Input: part model. Units: mm. Frame: model coordinates. A direction names the side the tool comes from. Round coordinates to 2 decimals unless told otherwise and drop trailing zeros. Order: outer loops, then holes, each group sorted by start corner. A loop starts at its lowest first (then second) coordinate and runs counter-clockwise, first axis right, second up. Notation, with made-up numbers: (85.5, -36.5) - (135.5, -36.5) arc R30 cw to (135.5, -0.5) - close; hole circle Ø8 at (-28.75, 16.5). An arc over 180 degrees is marked (long way). One line per item, written item: value. Start each with the question number.
Autodesk Inventor part; units mm, degrees
ref_plane "YZ Plane" through (0, 0, 0) normal (1, 0, 0) x (0, 1, 0)
ref_plane "XZ Plane" through (0, 0, 0) normal (0, 1, 0) x (-1, 0, 0)
ref_plane "XY Plane" through (0, 0, 0) normal (0, 0, 1) x (1, 0, 0)
sketch "Sketch1" plane through (0, 0, 0) normal (0, 0, 1) x (1, 0, 0)
  line L0 (20.5, -20.5) -> (20.5, -28.5)
  line L1 (28.5, -20.5) -> (20.5, -20.5)
  line L2 (28.5, 20.5) -> (28.5, -20.5)
  line L3 (20.5, 20.5) -> (28.5, 20.5)
  line L4 (20.5, 28.5) -> (20.5, 20.5)
  line L5 (-20.5, 28.5) -> (20.5, 28.5)
  line L6 (-20.5, 20.5) -> (-20.5, 28.5)
  line L7 (-28.5, 20.5) -> (-20.5, 20.5)
  line L8 (-28.5, -20.5) -> (-28.5, 20.5)
  line L9 (-20.5, -20.5) -> (-28.5, -20.5)
  line L10 (-20.5, -28.5) -> (-20.5, -20.5)
  line L11 (20.5, -28.5) -> (-20.5, -28.5)
  line L12 (-100, -100) -> (100, -100)
  line L13 (100, -100) -> (100, 100)
  line L14 (100, 100) -> (-100, 100)
  line L15 (-100, 100) -> (-100, -100)
  line L16 (-100, -100) -> (100, 100) construction
  line L17 (100, -100) -> (-100, 100) construction
  point P0 (0, 0)
  dimension "d0" = 200
  dimension "d1" = 200
extrude "Extrusion1" add sketch "Sketch1" along normal blind 8 contours L0 L11 L10 L9 L8 L7 L6 L5 L4 L3 L2 L1 | L15 L14 L13 L12
sketch "Sketch2" plane through (0, 0, 0) normal (0, 0, -1) x (-1, 0, 0)
  line L0 (28.5, -20.5) -> (28.5, 20.5)
  line L1 (28.5, 20.5) -> (20.5, 20.5)
  line L2 (20.5, 20.5) -> (20.5, 28.5)
  line L3 (20.5, 28.5) -> (-20.5, 28.5)
  line L4 (-20.5, 28.5) -> (-20.5, 20.5)
  line L5 (-20.5, 20.5) -> (-28.5, 20.5)
  line L6 (-28.5, 20.5) -> (-28.5, -20.5)
  line L7 (-28.5, -20.5) -> (-20.5, -20.5) construction
  line L8 (-20.5, -20.5) -> (-20.5, -28.5) construction
  line L9 (-28.5, -20.5) -> (-20.5, -20.5) construction
  line L10 (-28.5, -20.5) -> (-20.5, -20.5) construction
  line L11 (-20.5, -28.5) -> (20.5, -28.5) construction
  line L12 (20.5, -20.5) -> (28.5, -20.5)
  line L13 (20.5, -28.5) -> (20.5, -20.5)
  line L14 (-35, 35) -> (35, 35)
  line L15 (35, 35) -> (35, -35)
  line L16 (35, -35) -> (-35, -35)
  line L17 (-35, -35) -> (-35, 35)
  line L18 (-35, 35) -> (35, -35) construction
  line L19 (35, 35) -> (-35, -35) construction
  line L20 (-21, -29) -> (-21, -21)
  line L21 (-21, -21) -> (-29, -21)
  line L22 (-29, -21) -> (-29, 21)
  line L23 (-29, 21) -> (-21, 21)
  line L24 (-21, 21) -> (-21, 29)
  line L25 (-21, 29) -> (21, 29)
  line L26 (21, 29) -> (21, 21)
  line L27 (21, 21) -> (29, 21)
  line L28 (29, 21) -> (29, -21)
  line L29 (29, -21) -> (21, -21)
  line L30 (21, -21) -> (21, -29)
  line L31 (21, -29) -> (-21, -29)
  point P0 (0, 0)
  dimension "d4" = 70
  dimension "d5" = 70
  dimension "d6" = 0.5
extrude "Extrusion2" add sketch "Sketch2" along normal blind 35
sketch "Sketch3" plane through (0, 0, -35) normal (0, 0, -1) x (-1, 0, 0)
  line L0 (-35, -35) -> (35, -35)
  line L1 (35, -35) -> (35, 35)
  line L2 (35, 35) -> (-35, 35)
  line L3 (-35, 35) -> (-35, -35)
  line L4 (-21, -29) -> (-21, -21)
  line L5 (-21, -21) -> (-29, -21)
  line L6 (-29, -21) -> (-29, 21)
  line L7 (-29, 21) -> (-21, 21)
  line L8 (-21, 21) -> (-21, 29)
  line L9 (-21, 29) -> (21, 29)
  line L10 (21, 29) -> (21, 21)
  line L11 (21, 21) -> (29, 21)
  line L12 (29, 21) -> (29, -21)
  line L13 (29, -21) -> (21, -21)
  line L14 (21, -21) -> (21, -29)
  line L15 (21, -29) -> (-21, -29)
  line L16 (-29, 0) -> (-29, 10)
  line L17 (-29, -21) -> (-29, 21)
  line L18 (-29, 10) -> (-29, -10)
  line L19 (-29, 10) -> (-35, 10)
  line L20 (-35, 10) -> (-35, -10)
  line L21 (-35, -10) -> (-29, -10)
  line L22 (-29, -10) -> (-29, 10)
  point P0 (0, 0)
  dimension "d9" = 10
  dimension "d10" = 20
extrude "Extrusion3" cut sketch "Sketch3" against normal blind 35 contours L3 L19 L6 L21
chamfer "Chamfer1" distance 19.4625 angle 45 5 edges at (35, 22.5, 0) (35, -22.5, 0) (0, -35, 0) (-35, 0, 0) (0, 35, 0)
sketch "Sketch4" plane through (0, 0, -35) normal (0, 0, -1) x (-1, 0, 0)
  circle A0 centre (24.5, 24.5) radius 2.5
  circle A1 centre (24.5, -24.5) radius 2.5
  circle A2 centre (-24.5, -24.5) radius 2.5
  circle A3 centre (-24.5, 24.5) radius 2.5
  circle A4 centre (24.5, 24.5) radius 3
  circle A5 centre (-24.5, 24.5) radius 3
  circle A6 centre (-24.5, -24.5) radius 3
  circle A7 centre (24.5, -24.5) radius 3
  point P0 (0, 0)
  dimension "d16" = 6
  dimension "d17" = 6
  dimension "d18" = 6
  dimension "d19" = 6
extrude "Extrusion4" cut sketch "Sketch4" against normal blind 10 contours A0 | A1 | A2 | A3 | A4 | A5 | A6 | A7
fillet "Fillet1" radius 2 4 edges at (100, 100, 4) (100, -100, 4) (-100, -100, 4) (-100, 100, 4)
properties part number "Base stand"
1. Pin query (flat end, axial travel): pin 1 (12 mm diameter, centred on x = 42, y = -39, fed in from -Z); pin 2 (8 mm diameter, centred on y = -55.5, z = -1.5, fed in from +X); pin 3 (10.5 mm diameter, centred on x = -1.5, z = -13, fed in from -Y); pin 4 (4 mm diameter, centred on x = -45.5, z = -4.5, fed in from +Y). Return the tip coordinate at first contact, or that it passes through.
2. Set-up query: faces 1 (the face through (-44.595, -0.762, -9.867)), 2 (the face through (36, -10, -14)), 3 (the face through (-21, 25, -17)), 4 (the face through (-1, -100, 4)), 5 (the face through (35, 22, -27)). Return all of +Z, -Z, +X, -X, +Y, -Y with unobstructed straight access to the full face (end or side cutting, diameter ignored); none if empty.
3. Section C-C (y = -24.5). Return the cut outline in (x, z), then the cut area to 3 significant figures.
4. Section B-B (z = -28.5). Return the cut outline in (x, y), then the cut area to 3 significant figures.
5. Line query: line 1 (X direction, y = 24, z = -29); line 2 (Y direction, x = -24.5, z = -28); line 3 (Y direction, x = -14, z = -24). Output: solid intervals per line, ascending. Write a range as from..to.
6. Section A-A (x = 7.5). Return the cut outline in (y, z), then the cut area to 3 significant figures.
7. Pull-direction query (Y, two-part tool) for faces 6 (the face through (-35, 0, -27)), 7 (the face through (-25, 21, -17)), 8 (the face through (0.762, -44.595, -9.867)); classes: released by +Y, released by -Y, zero draft, split by the parting line, or undercut.
8. Section D-D (z = -11). Return the cut outline in (x, y), then the cut area to 3 significant figures.
Solved:
1. pin 1: stops at z = -17.93
1. pin 2: stops at x = 100
1. pin 3: stops at y = -46.71
1. pin 4: stops at y = 51.96
2. face 1: -Z, -X, +Y, -Y
2. face 2: -Z, +X
2. face 3: -Z
2. face 4: +Z, -Z, +X, -X, -Y
2. face 5: -Z, +X, +Y, -Y
3. outline: (-100, 0) - (-54.46, 0) - (-35, -19.46) - (-35, -35) - (-27.5, -35) - (-27.5, -25) - (-21.5, -25) - (-21.5, -35) - (-21, -35) - (-21, 0) - (21, 0) - (21, -35) - (21.5, -35) - (21.5, -25) - (27.5, -25) - (27.5, -35) - (35, -35) - (35, -19.46) - (54.46, 0) - (100, 0) - (100, 8) - (-100, 8) - close
3. area: 2,840 mm²
4. outline: (-35, -35) - (35, -35) - (35, -10) - (29, -10) - (29, -21) - (21, -21) - (21, -29) - (-21, -29) - (-21, -21) - (-29, -21) - (-29, 21) - (-21, 21) - (-21, 29) - (21, 29) - (21, 21) - (29, 21) - (29, 10) - (35, 10) - (35, 35) - (-35, 35) - close; hole circle Ø6 at (-24.5, -24.5); hole circle Ø6 at (-24.5, 24.5); hole circle Ø6 at (24.5, -24.5); hole circle Ø6 at (24.5, 24.5)
4. area: 1,560 mm²
5. line 1: x = -35..-27.46, -21.54..-21, 21..21.54, 27.46..35
5. line 2: y = -35..-27.5, -21.5..-21, 21..21.5, 27.5..35
5. line 3: y = -35..-29, 29..35
6. outline: (-100, 0) - (-54.46, 0) - (-35, -19.46) - (-35, -35) - (-29, -35) - (-29, 0) - (29, 0) - (29, -35) - (35, -35) - (35, -19.46) - (54.46, 0) - (100, 0) - (100, 8) - (-100, 8) - close
6. area: 2,400 mm²
7. face 6: zero draft
7. face 7: undercut
7. face 8: released by -Y
8. outline: (-43.46, -43.46) - (43.46, -43.46) - (43.46, -10) - (29, -10) - (29, -21) - (21, -21) - (21, -29) - (-21, -29) - (-21, -21) - (-29, -21) - (-29, 21) - (-21, 21) - (-21, 29) - (21, 29) - (21, 21) - (29, 21) - (29, 10) - (43.46, 10) - (43.46, 43.46) - (-43.46, 43.46) - close
8. area: 4,160 mm²
